Here's how the part is built. I have some questions about the finished solid (model axes, mm). Face numbers are marked on the shaded views. A direction names the side the tool comes from. Give positions to 0.01 mm unless a question says otherwise; leave off trailing zeros. Loops run counter-clockwise (first coordinate to the right, second up) from the corner with the lowest first, then second, coordinate; pieces in that order, holes last.
Q1. Suppose I cut it at D-D (y = 45). List the corners of the cut face in (x, z) for me.
Q2. Suppose I cut it at B-B (x = 0). List the corners of the cut face in (y, z) for me, and give its area (3 significant figures).
Q3. I'm going to push flat-ended pins straight in: P1, Ø4, axis at x = 9, z = 0.5, coming from the -Y side; P2, Ø2.5, axis at x = -11.11, z = -12.7, coming from the -Y side; P3, Ø1.5, axis at x = 4, z = 5.5, coming from the -Y side. Where does each tip first touch, or does it pass through?
Q4. I need wall thicknesses on probe 1 along Z at (x, y) = (0, 59); probe 2 along Z at (x, y) = (-9.5, 14); probe 3 along Z at (x, y) = (0, 34). Which ranges of each line are inside material? Lowest first, please.
Q5. Suppose I cut it at A-A (z = 0). List the corners of the cut face in (x, y) for me.
Q6. Thinking about a two-plate mould opening in Y: for the marked faces 1, 2 and 3, which applies, pulls with the +Y half, pulls with the -Y half, needs draft (parallel to the pull), parting line crosses it, or undercut?
Q7. For the marked faces 4 and 5, which set-ups out of +Z, -Z, +X, -X, +Y, -Y let a thin tool reach every point of the face, with its end or its side?
Q8. Suppose I cut it at C-C (y = 17). List the corners of the cut face in (x, z) for me, and give its area (3 significant figures).
```python
from build123d import *

# Parameters (mm, degrees)
SKETCH1_W                  = 50.8
SKETCH1_H                  = 50.8
BLOCK_DEPTH                = 60.96
SPRING_BORE_D              = 25.4
SPRING_BORE_DEPTH          = 50.292
SPRING_BORE_TIP            = 7.630929862
F_1_2_20_TAPPED_HOLE_D     = 11.50874
F_10_32_TAPPED_HOLES_D     = 4.0386
F_10_32_TAPPED_HOLES_DEPTH = 19.05
F_10_32_TAPPED_HOLES_TIP   = 1.213317848
VIEW_HOLE_D                = 7.9375


with BuildPart() as part:
    # Sketch1 → Block (new body)
    with BuildSketch(Plane(origin=(0, 0, 0), x_dir=(1, 0, 0), z_dir=(0, 1, 0))):
        Rectangle(SKETCH1_W, SKETCH1_H)
    extrude(amount=BLOCK_DEPTH)

    # Spring Bore
    with Locations(Plane(origin=(0, 0, 0), x_dir=(-1, 0, 0), z_dir=(0, -1, 0))):
        with Locations((0, 0)):
            Hole(SPRING_BORE_D / 2, depth=SPRING_BORE_DEPTH)
            with Locations((0, 0, -(SPRING_BORE_DEPTH + SPRING_BORE_TIP / 2))):  # 118° drill point
                Cone(0, SPRING_BORE_D / 2, SPRING_BORE_TIP, mode=Mode.SUBTRACT)

    # 1/2-20 Tapped Hole (through all)
    with Locations(Plane(origin=(0, 60.96, 0), x_dir=(1, 0, 0), z_dir=(0, 1, 0))):
        with Locations((0, 0)):
            Hole(F_1_2_20_TAPPED_HOLE_D / 2)

    # #10-32 Tapped Holes
    with Locations(Plane(origin=(0, 0, 0), x_dir=(-1, 0, 0), z_dir=(0, -1, 0))):
        with Locations((11.1125, 12.7), (11.1125, -12.7), (-11.1125, -12.7), (-11.1125, 12.7), (0, 0)):
            Hole(F_10_32_TAPPED_HOLES_D / 2, depth=F_10_32_TAPPED_HOLES_DEPTH)
            with Locations((0, 0, -(F_10_32_TAPPED_HOLES_DEPTH + F_10_32_TAPPED_HOLES_TIP / 2))):  # 118° drill point
                Cone(0, F_10_32_TAPPED_HOLES_D / 2, F_10_32_TAPPED_HOLES_TIP, mode=Mode.SUBTRACT)

    # View Hole (through all)
    with Locations(Plane.XY.offset(25.4)):
        with Locations((0, 50.292)):
            Hole(VIEW_HOLE_D / 2)


solid = part.part
```
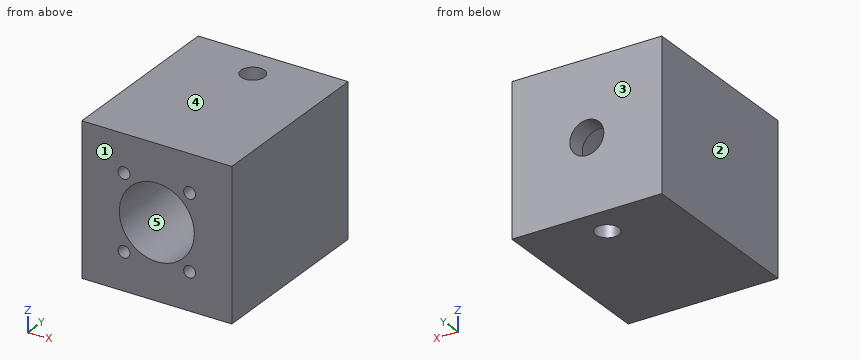
Solutions:
1. outline: (-25.4, -25.4) - (25.4, -25.4) - (25.4, 25.4) - (-25.4, 25.4) - close; hole circle Ø25.4 at (0, 0)
2. outline: (0, -25.4) - (46.32, -25.4) - (46.32, -12.7) - (0, -12.7) - close; (0, 12.7) - (46.32, 12.7) - (46.32, 25.4) - (0, 25.4) - close; (54.26, -25.4) - (60.96, -25.4) - (60.96, -5.75) - (54.47, -5.75) - (54.26, -6.09) - close; (54.26, 6.09) - (54.47, 5.75) - (60.96, 5.75) - (60.96, 25.4) - (54.26, 25.4) - close
2. area: 1,440 mm2
3. P1: stops at y = 51.31
3. P2: stops at y = 19.51
3. P3: stops at y = 53.39
4. probe 1: z = -25.4 to -5.75, 5.75 to 25.4
4. probe 2: z = -25.4 to -13.92, -11.48 to -8.43, 8.43 to 11.48, 13.92 to 25.4
4. probe 3: z = -25.4 to -12.7, 12.7 to 25.4
5. outline: (-25.4, 0) - (-12.7, 0) - (-12.7, 50.29) - (-5.75, 54.47) - (-5.75, 60.96) - (-25.4, 60.96) - close; (5.75, 54.47) - (12.7, 50.29) - (12.7, 0) - (25.4, 0) - (25.4, 60.96) - (5.75, 60.96) - close
6. face 1: pulls with the -Y half
6. face 2: needs draft
6. face 3: pulls with the +Y half
7. face 4: +Z, +X, -X, +Y, -Y
7. face 5: -Y
8. outline: (-25.4, -25.4) - (25.4, -25.4) - (25.4, 25.4) - (-25.4, 25.4) - close; hole circle Ø4.04 at (-11.11, -12.7); hole circle Ø4.04 at (-11.11, 12.7); hole circle Ø25.4 at (0, 0); hole circle Ø4.04 at (11.11, -12.7); hole circle Ø4.04 at (11.11, 12.7)
8. area: 2,020 mm2
